from build123d import *

# Parameters (mm, degrees)
F0_W     = 127
F0_H     = 76.2
F1_DEPTH = 12.7
F2_R     = 6.35
F3_DEPTH = 12.701
F4_SIZE  = 2.54
F7_R     = 2.53999
F8_SIZE  = 2.54


# Not quite as in the source:
# - a fillet or chamfer is up to 0.001 mm smaller than in the source, because OpenCascade refuses the exact size


with BuildPart() as f1:
    # F0 (on Top) → F1 (new body)
    with BuildSketch(Plane.XY):
        Rectangle(F0_W, F0_H)
    extrude(amount=F1_DEPTH)

    # F2 (on face) → F3 (cut, through all)
    with BuildSketch(Plane.XY.offset(12.7)):
        with Locations((-44.45, 19.05)):
            Circle(F2_R)
        with Locations((44.45, 19.05)):
            Circle(F2_R)
        with Locations((44.45, -19.05)):
            Circle(F2_R)
        with Locations((-44.45, -19.05)):
            Circle(F2_R)
    extrude(amount=-F3_DEPTH, mode=Mode.SUBTRACT)

    # F4
    f4_edges = [f1.edges().sort_by_distance(p)[0] for p in [
        (-63.5, 0, 12.7),
        (0, 38.1, 12.7),
        (0, -38.1, 12.7),
        (63.5, 0, 12.7),
    ]]
    chamfer(f4_edges, length=F4_SIZE)

    # F5 (on Front) → F6 (revolve)
    with BuildSketch(Plane.XZ):
        Polygon((0, 38.1), (0, 12.7), (12.7, 12.7), (12.7, 22.86), (8.3547569811, 22.86), (8.3547569811, 27.94), (12.7, 27.94), (12.7, 38.1), align=None)
    revolve(axis=Axis((0, 0, 25.4), (0, 0, 1)))

    # F7 (radius 2.54 in the source; OpenCascade refuses exactly that, so slightly less here)
    f7_edges = [f1.edges().sort_by_distance(p)[0] for p in [
        (-12.7, 0, 12.7),
        (-8.354757, 0, 22.86),
        (-8.354757, 0, 27.94),
    ]]
    fillet(f7_edges, radius=F7_R)

    # F8
    f8_edges = [f1.edges().sort_by_distance(p)[0] for p in [
        (-12.7, 0, 38.1),
    ]]
    chamfer(f8_edges, length=F8_SIZE)


solid = f1.part
Source: CAD feature listing. Evaluate the final solid. Frame: model axes, mm. A direction names the side the tool comes from. Round coordinates to 2 decimals unless told otherwise and drop trailing zeros. Loops run counter-clockwise (first coordinate to the right, second up) from the corner with the lowest first, then second, coordinate; pieces in that order, holes last. Notation, with made-up numbers: (-27, -0.5) - (6, -0.5) arc R24 cw to (6, 35.5) - close; hole circle Ø8 at (80.5, -39.75). An arc over 180 degrees is marked (long way). Write item = value, one per line. Start each with the question number.
(1) Set-up query: faces 1 (the face through (-1, 16, 12.7)), 2 (the face through (-1, -38.1, 5)). Return all of +Z, -Z, +X, -X, +Y, -Y with unobstructed straight access to the full face (end or side cutting, diameter ignored); none if empty.
(2) Section query B-B, the plane x = -44.45. Output: boundary loops of the cut face in (y, z).
(3) Pin query (flat end, axial travel): pin 1 (1.5 mm diameter, centred on x = 12.5, y = 15.5, fed in from +Z); pin 2 (10 mm diameter, centred on x = 48.5, z = 21, fed in from +Y); pin 3 (12 mm diameter, centred on y = -6.5, z = 30, fed in from -X); pin 4 (8 mm diameter, centred on y = -9, z = 22.5, fed in from -X). Return the tip coordinate at first contact, or that it passes through.
(4) Ray query, line 1 along Y through (x, z) = (-44, 5); line 2 along X through (y, z) = (-19, 4); line 3 along Y through (x, z) = (46.5, 12). Return the intervals inside material, ascending. Write a range as from..to.
(5) Pull-direction query (Z, two-part tool) for faces 3 (the face through (63.5, -1, 5)), 4 (the face through (0, 0, 38.1)), 5 (the face through (-3.7, 10.41, 27.94)), 6 (the face through (3.7, 10.41, 22.86)); classes: +Z half, -Z half, draft (parallel to the pull), parting line (faces both ways), or undercut.
(6) Section query A-A, the plane y = -19.05. Output: boundary loops of the cut face in (x, z).
(7) Section query C-C, the plane z = 7. Output: boundary loops of the cut face in (x, y), plus the area to 3 significant figures.
Conclusion:
q1.face_1 = +Z
q1.face_2 = +Z, -Z, +X, -X, -Y
q2.outline = (-38.1, 0) - (-25.4, 0) - (-25.4, 12.7) - (-35.56, 12.7) - (-38.1, 10.16) - close; (-12.7, 0) - (12.7, 0) - (12.7, 12.7) - (-12.7, 12.7) - close; (25.4, 0) - (38.1, 0) - (38.1, 10.16) - (35.56, 12.7) - (25.4, 12.7) - close
q3.pin_1 = 12.7
q3.pin_2 = through
q3.pin_3 = -12.69
q3.pin_4 = -11.67
q4.line_1 = -38.1..-25.38, -12.72..12.72, 25.38..38.1
q4.line_2 = -63.5..-50.8, -38.1..38.1, 50.8..63.5
q4.line_3 = -36.26..-25.06, -13.04..13.04, 25.06..36.26
q5.face_3 = draft
q5.face_4 = +Z half
q5.face_5 = undercut
q5.face_6 = undercut
q6.outline = (-63.5, 0) - (-50.8, 0) - (-50.8, 12.7) - (-60.96, 12.7) - (-63.5, 10.16) - close; (-38.1, 0) - (38.1, 0) - (38.1, 12.7) - (-38.1, 12.7) - close; (50.8, 0) - (63.5, 0) - (63.5, 10.16) - (60.96, 12.7) - (50.8, 12.7) - close
q7.outline = (-63.5, -38.1) - (63.5, -38.1) - (63.5, 38.1) - (-63.5, 38.1) - close; hole circle Ø12.7 at (-44.45, -19.05); hole circle Ø12.7 at (-44.45, 19.05); hole circle Ø12.7 at (44.45, -19.05); hole circle Ø12.7 at (44.45, 19.05)
q7.area = 9,170 mm2
